Verification items for the finished model (mm, model axes). A direction names the side the tool comes from. Round coordinates to 2 decimals unless told otherwise and drop trailing zeros. Order: outer loops, then holes, each group sorted by start corner. A loop starts at its lowest first (then second) coordinate and runs counter-clockwise, first axis right, second up. Notation, with made-up numbers: (84.25, -29) -> (101.25, -29) arc R30 ccw to (101.25, 0) -> close; hole circle Ø8 at (-23, 18.5). An arc over 180 degrees is marked (long way). Put each result on its own line as item: value.
from build123d import *

# Parameters (mm, degrees)
SKETCH1_W                    = 150
SKETCH1_H                    = 150
BASE_FLANGE1_DEPTH           = 3
EDGE_FLANGE1_STRIP_W         = 13.4732
EDGE_FLANGE1_STRIP_H         = 3
EDGE_FLANGE1_STRIP_CUT_DEPTH = 150
EDGE_FLANGE1_DEPTH           = 150
EDGE_FLANGE2_STRIP_W         = 13.4732
EDGE_FLANGE2_STRIP_H         = 3
EDGE_FLANGE2_STRIP_CUT_DEPTH = 150
EDGE_FLANGE2_DEPTH           = 150
CUT_EXTRUDE1_DEPTH           = 10


# Sheet-metal steps are written as plain solids
with BuildPart() as part:
    # Sketch1 → Base-Flange1 (new body)
    with BuildSketch(Plane(origin=(0, 0, 0), x_dir=(1, 0, 0), z_dir=(0, 1, 0))):
        with Locations((-55.705035971, -46.04676259)):
            Rectangle(SKETCH1_W, SKETCH1_H)
        with BuildLine():
            Line((-101.705035971, 4.95323741), (-101.705035971, -97.04676259))
            ThreePointArc((-101.705035971, -97.04676259), (-105.705035971, -101.04676259), (-109.705035971, -97.04676259))
            Line((-109.705035971, -97.04676259), (-109.705035971, 4.95323741))
            ThreePointArc((-109.705035971, 4.95323741), (-105.705035971, 8.95323741), (-101.705035971, 4.95323741))
        make_face(mode=Mode.SUBTRACT)
        with BuildLine():
            Line((-1.705035971, 4.95323741), (-1.705035971, -97.04676259))
            ThreePointArc((-1.705035971, -97.04676259), (-5.705035971, -101.04676259), (-9.705035971, -97.04676259))
            Line((-9.705035971, -97.04676259), (-9.705035971, 4.95323741))
            ThreePointArc((-9.705035971, 4.95323741), (-5.705035971, 8.95323741), (-1.705035971, 4.95323741))
        make_face(mode=Mode.SUBTRACT)
    extrude(amount=-BASE_FLANGE1_DEPTH)

    # Edge-Flange1 strip (across the edge) → Edge-Flange1 strip cut (cut)
    with BuildSketch(Plane(origin=(19.294964029, 0, -28.95323741), x_dir=(0, 0, 1), z_dir=(-1, 0, 0))):
        with Locations((-3, -1.5)):
            Rectangle(EDGE_FLANGE1_STRIP_W, EDGE_FLANGE1_STRIP_H)
    extrude(amount=EDGE_FLANGE1_STRIP_CUT_DEPTH, mode=Mode.SUBTRACT)

    # Edge-Flange1 section (across the edge) → Edge-Flange1 (add)
    with BuildSketch(Plane(origin=(19.294964029, 0, -28.95323741), x_dir=(0, 0, 1), z_dir=(-1, 0, 0))):
        with BuildLine():
            Line((0, 0.7366), (0, 167))
            Line((0, 167), (3, 167))
            Line((3, 167), (3, 0.7366))
            ThreePointArc((3, 0.7366), (3.215745145, 0.215745145), (3.7366, 0))
            Line((3.7366, 0), (3.7366, -3))
            ThreePointArc((3.7366, -3), (1.094424801, -1.905575199), (0, 0.7366))
        make_face()
    extrude(amount=EDGE_FLANGE1_DEPTH)

    # Edge-Flange2 strip (across the edge) → Edge-Flange2 strip cut (cut)
    with BuildSketch(Plane(origin=(19.294964029, 167, -25.95323741), x_dir=(0, -1, 0), z_dir=(-1, 0, 0))):
        with Locations((-3, -1.5)):
            Rectangle(EDGE_FLANGE2_STRIP_W, EDGE_FLANGE2_STRIP_H)
    extrude(amount=EDGE_FLANGE2_STRIP_CUT_DEPTH, mode=Mode.SUBTRACT)

    # Edge-Flange2 section (across the edge) → Edge-Flange2 (add)
    with BuildSketch(Plane(origin=(19.294964029, 167, -25.95323741), x_dir=(0, -1, 0), z_dir=(-1, 0, 0))):
        with BuildLine():
            Line((0, 0.7366), (0, 32))
            Line((0, 32), (3, 32))
            Line((3, 32), (3, 0.7366))
            ThreePointArc((3, 0.7366), (3.215745145, 0.215745145), (3.7366, 0))
            Line((3.7366, 0), (3.7366, -3))
            ThreePointArc((3.7366, -3), (1.094424801, -1.905575199), (0, 0.7366))
        make_face()
    extrude(amount=EDGE_FLANGE2_DEPTH)

    # Sketch12 → Cut-Extrude1 (cut)
    with BuildSketch(Plane(origin=(0, 167, 0), x_dir=(1, 0, 0), z_dir=(0, 1, 0))):
        with BuildLine():
            Line((4.294964029, 4.95323741), (-15.705035971, 4.95323741))
            ThreePointArc((-15.705035971, 4.95323741), (-19.705035971, 8.95323741), (-15.705035971, 12.95323741))
            Line((-15.705035971, 12.95323741), (4.294964029, 12.95323741))
            ThreePointArc((4.294964029, 12.95323741), (8.294964029, 8.95323741), (4.294964029, 4.95323741))
        make_face()
        with BuildLine():
            Line((-115.705035971, 4.95323741), (-97.680274897, 4.95323741))
            ThreePointArc((-97.680274897, 4.95323741), (-93.680274897, 8.95323741), (-97.680274897, 12.95323741))
            Line((-97.680274897, 12.95323741), (-115.705035971, 12.95323741))
            ThreePointArc((-115.705035971, 12.95323741), (-119.705035971, 8.95323741), (-115.705035971, 4.95323741))
        make_face()
    extrude(amount=-CUT_EXTRUDE1_DEPTH, mode=Mode.SUBTRACT)


solid = part.part
Item 1: Section check B-B on x = -23.5. Record the boundary of the cut face in (y, z).
Check sheet entries:
outline: (-3, -25.22) arc R3.74 ccw to (0.74, -28.95) -> (163.26, -28.95) arc R3.74 ccw to (167, -25.22) -> (167, 6.05) -> (164, 6.05) -> (164, -25.22) arc R0.74 cw to (163.26, -25.95) -> (0.74, -25.95) arc R0.74 cw to (0, -25.22) -> (0, 121.05) -> (-3, 121.05) -> close
Item 2: Tool access check on faces 1 (the flat face through (-57, 0, 47)), 2 (the flat face through (-55, 81, -28.953)). Record the directions out of +Z, -Z, +X, -X, +Y, -Y that give a thin tool (end or side, any length) a straight path to the whole face; none if there is none.
Check sheet entries:
face 1: +Z, +X, -X
face 2: -Z, +X, -X, +Y, -Y
Item 3: Section check A-A on z = 34. Record the boundary of the cut face in (x, y).
Check sheet entries:
outline: (-130.71, -3) -> (-109.71, -3) -> (-109.71, 0) -> (-130.71, 0) -> close; (-101.71, -3) -> (-9.71, -3) -> (-9.71, 0) -> (-101.71, 0) -> close; (-1.71, -3) -> (19.29, -3) -> (19.29, 0) -> (-1.71, 0) -> close
Item 4: Release check for a two-part mould opening along Y. For faces 3 (the flat face through (19.295, -0.2, 46.4)), 4 (the flat face through (-55, 83, -25.953)), 5 (the flat face through (-55, 167, -10)) record: +Y half, -Y half, draft (parallel to the pull), parting line (faces both ways), or undercut.
Check sheet entries:
face 3: draft
face 4: undercut
face 5: +Y half
Item 5: Gauge pin test, flat ends, axial feed: pin 1 Ø3.5 at (x, y) = (-1.5, 165.5) entering from -Z; pin 2 Ø0.9 at (x, y) = (-111, 165.5) entering from +Z; pin 3 Ø5 at (x, z) = (-8, 5) entering from -Y; pin 4 Ø0.9 at (x, y) = (-106.5, 165.5) entering from -Z. Record the tip position at first contact, or that the pin passes through.
Check sheet entries:
pin 1: stops at z = -28.92
pin 2: stops at z = 6.05
pin 3: stops at y = -3
pin 4: stops at z = -28.5
Item 6: Material ranges on L1, parallel to Y at x = -114.5, z = -2; L2, parallel to Z at x = -105, y = 122.5; L3, parallel to Y at x = -65.5, z = 83, recorded low to high. Write a range as [from, to].
Check sheet entries:
L1: y = [-3, 0], [164, 167]
L2: z = [-28.95, -25.95]
L3: y = [-3, 0]
Item 7: Section check C-C on y = 29.5. Record the boundary of the cut face in (x, z).
Check sheet entries:
outline: (-130.71, -28.95) -> (19.29, -28.95) -> (19.29, -25.95) -> (-130.71, -25.95) -> close
